from build123d import *

# Parameters (mm, degrees)
SKETCH_W        = 50
SKETCH_H        = 50
PAD_DEPTH       = 8
SKETCH001_R     = 20
PAD001_DEPTH    = 10
SKETCH002_R     = 17.994409
POCKET_DEPTH    = 18.001
SKETCH003_W     = 45
SKETCH003_H     = 3
POCKET001_DEPTH = 43


with BuildPart() as part:
    # Sketch → Pad (new body)
    with BuildSketch(Plane.XY):
        Rectangle(SKETCH_W, SKETCH_H)
    extrude(amount=PAD_DEPTH)

    # Sketch001 → Pad001 (new body)
    with BuildSketch(Plane.XY.offset(8)):
        Circle(SKETCH001_R)
    extrude(amount=PAD001_DEPTH)

    # Sketch002 → Pocket (cut, through all)
    with BuildSketch(Plane.XY.offset(18)):
        Circle(SKETCH002_R)
    extrude(amount=-POCKET_DEPTH, mode=Mode.SUBTRACT)

    # Sketch003 → Pocket001 (cut)
    with BuildSketch(Plane.XZ.offset(25)):
        with Locations((0, 4)):
            Rectangle(SKETCH003_W, SKETCH003_H)
    extrude(amount=-POCKET001_DEPTH, mode=Mode.SUBTRACT)


solid = part.part
Geometry: final body of the model. Coordinates: model frame, mm. A direction names the side the tool comes from. Give positions to 0.01 mm unless a question says otherwise; leave off trailing zeros. Write each loop counter-clockwise with the first axis right and the second up, starting at its lowest first coordinate (ties: lowest second). Pieces come first, ordered by that corner, then holes. Notation, with made-up numbers: (40, 1.25) - (95, 1.25) arc R33 ccw to (95, 32.25) - close; hole circle Ø3 at (-15, 47). An arc over 180 degrees is marked (long way). Return JSON: item names as keys, results as strings. Group by question number.
1) Mould query, pull axis Y, two halves, no side actions, for faces 1 (the cylindrical face through (-3.901, -17.567, 1.267)), 2 (the flat face through (-18, 3, 18)), 3 (the cylindrical face through (-3.901, -17.567, 11.838)), 4 (the flat face through (0, 25, 4)). Classes: released by +Y, released by -Y, zero draft, split by the parting line, or undercut.
2) Section C-C on z = 14. Return the cut outline in (x, y).
3) Section D-D on y = 8. Return the cut outline in (x, z), plus the area to 3 significant figures.
4) Section A-A on x = 0. State how many separate pieces and enclosed holes the cut face has, plus the area to 3 significant figures.
5) First-contact query: P1, Ø1.5, axis at x = -6, z = 8.5, coming from the -Y side; P2, Ø6, axis at x = 16, y = -19.5, coming from the +Z side; P3, Ø2.5, axis at x = -4, z = 4, coming from the -Y side; P4, Ø12, axis at x = -10.5, y = -2, coming from the +Z side. Flat tips, straight axial feed; report the tip coordinate or a pass-through.
6) Line query: line 1 (Z direction, x = -21, y = 0); line 2 (X direction, y = -18, z = 4.5); line 3 (Z direction, x = -5, y = -17.5). Output: solid intervals per line, ascending.
7) Section B-B on y = 0. Return the cut outline in (x, z).
8) Set-up query: faces 5 (the flat face through (0, 18, 4)), 6 (the cylindrical face through (-4.336, -19.524, 12.93)), 7 (the flat face through (-11, 17, 0)). Return all of +Z, -Z, +X, -X, +Y, -Y with unobstructed straight access to the full face (end or side cutting, diameter ignored); none if empty.
Filled in:
{
 "1": {"face 1": "undercut", "face 2": "zero draft", "face 3": "undercut", "face 4": "released by +Y"},
 "2": {"outline": "circle Ø40 at (0, 0); hole circle Ø35.99 at (0, 0)"},
 "3": {"outline": "(-25, 0) - (-16.12, 0) - (-16.12, 2.5) - (-22.5, 2.5) - (-22.5, 5.5) - (-16.12, 5.5) - (-16.12, 18) - (-18.33, 18) - (-18.33, 8) - (-25, 8) - close; (16.12, 0) - (25, 0) - (25, 8) - (18.33, 8) - (18.33, 18) - (16.12, 18) - (16.12, 5.5) - (22.5, 5.5) - (22.5, 2.5) - (16.12, 2.5) - close", "area": "148 mm^2"},
 "4": {"separate pieces": "3", "enclosed holes": "0", "area": "131 mm^2"},
 "5": {"P1": "stops at y = -25", "P2": "stops at z = 8", "P3": "stops at y = 18", "P4": "passes through"},
 "6": {"line 1": "z = 0 to 2.5, 5.5 to 8", "line 2": "x = -25 to -22.5, 22.5 to 25", "line 3": "z = 0 to 2.5, 5.5 to 18"},
 "7": {"outline": "(-25, 0) - (-17.99, 0) - (-17.99, 2.5) - (-22.5, 2.5) - (-22.5, 5.5) - (-17.99, 5.5) - (-17.99, 18) - (-20, 18) - (-20, 8) - (-25, 8) - close; (17.99, 0) - (25, 0) - (25, 8) - (20, 8) - (20, 18) - (17.99, 18) - (17.99, 5.5) - (22.5, 5.5) - (22.5, 2.5) - (17.99, 2.5) - close"},
 "8": {"face 5": "-Y", "face 6": "+Z", "face 7": "-Z, +X, -X, +Y, -Y"}
}
